Geometry: final body of the model. Coordinates: model frame, mm. A direction names the side the tool comes from. Give positions to 0.01 mm unless a question says otherwise; leave off trailing zeros. Loops run counter-clockwise (first coordinate to the right, second up) from the corner with the lowest first, then second, coordinate; pieces in that order, holes last.
1. Access query for faces 4 (the face through (53.24, -0.53, -11.99)), 5 (the face through (4.93, -18.17, 24.53)), 6 (the face through (135.357, 87.741, -3.252)), 7 (the face through (145.386, 68.872, -41.002)). Directions: +Z, -Z, +X, -X, +Y, -Y. A direction counts if a zero-diameter tool reaches every point of the face in a straight line with its end or side. Return the directions, or none.
2. Material intervals for line 1 along X through (y, z) = (108, 0); line 2 along Z through (x, y) = (70, 0); line 3 along Z through (x, y) = (210, 176), sorted ascending.
3. Section A-A, the plane y = 60. Output: boundary loops of the cut face in (x, z), then the cut area to 3 significant figures.
4. Draft query along Y for faces 1 (the face through (0, -8.3, 9.4)), 2 (the face through (238.394, 189.798, 141.033)), 3 (the face through (224.07, 177.95, 140.47)). Return one class per face: +Y half, -Y half, draft (parallel to the pull), parting line (faces both ways), or undercut.
5. First-contact query: P1, Ø19, axis at x = 150, z = 0, coming from the -Y side; P2, Ø3, axis at x = 153, z = -25.5, coming from the +Y side; P3, Ø14.5, axis at y = 0, z = 0, coming from the -X side. Flat tips, straight axial feed; report the tip coordinate or a pass-through.
from build123d import *

# Parameters (mm, degrees)
SWEEP_2_PROFILE_R    = 15
SWEEP_6_PROFILE_R    = 15
SKETCH_7_R           = 40
EXTRUDE_2_DEPTH      = 10
SKETCH_8_R           = 4.5
CUT_EXTRUDE_1_DEPTH  = 357.575052533
SWEEP_START          = 287.981272568
SWEEP_8_OUTLINE_R    = 45
SWEEP_8_DEPTH        = 12.094233032
SWEEP_START_2        = 300
SWEEP_8_2_OUTLINE_W  = 93
SWEEP_8_2_OUTLINE_H  = 93
SWEEP_8_2_DEPTH      = 1
EXTRUDE_3_REACH      = 435.125
EXTRUDE_3_END_RADIUS = 15
SKETCH_15_R          = 10
SWEEP_2_2_PROFILE_R  = 12
SWEEP_4_PROFILE_R    = 12
SKETCH_19_R          = 7
CUT_EXTRUDE_2_DEPTH  = 70
SWEEP_14_PROFILE_R   = 5.5
SWEEP_16_PROFILE_R   = 5.5
SWEEP_18_PROFILE_R   = 5.5
SWEEP_20_PROFILE_R   = 5.5


with BuildPart() as part:
    # Sweep 2: sweep along a path in 草图1
    with BuildLine(Plane.XY) as sweep_2_path:
        Line((0, 0), (105, 0))
        ThreePointArc((105, 0), (136.819805153, 13.180194847), (150, 45))
        Line((150, 45), (150, 77.56))
    # Sweep 2 profile (on start of the path) → Sweep 2 (sweep)
    with BuildSketch(Plane(origin=(0, 0, 0), x_dir=(0, 0, 1), z_dir=(1, 0, 0))):
        Circle(SWEEP_2_PROFILE_R)
    sweep(path=sweep_2_path.line)

    # 扫描6: sweep along a curve in space
    with BuildLine() as sweep_6_path:
        Line((150, 50, 0), (150, 120, 0))
        Line((150, 120, 0), (230, 200, 140))
    # 扫描6 profile (on start of the path) → 扫描6 (sweep)
    with BuildSketch(Plane(origin=(150, 50, 0), x_dir=(0, 0, 1), z_dir=(0, 1, 0))):
        Circle(SWEEP_6_PROFILE_R)
    sweep(path=sweep_6_path.line, transition=Transition.RIGHT)

    # 草图7 → 凸台-拉伸2 (add)
    with BuildSketch(Plane(origin=(0, 0, 0), x_dir=(0, 0, -1), z_dir=(1, 0, 0))):
        Circle(SKETCH_7_R)
    extrude(amount=EXTRUDE_2_DEPTH)

    # 草图8 → 切除-拉伸1 (cut, through all)
    with BuildSketch(Plane(origin=(0, 0, 0), x_dir=(0, 0, -1), z_dir=(1, 0, 0))):
        with Locations((-21.213203, 21.213203)):
            Circle(SKETCH_8_R)
        with Locations((21.213203, 21.213203)):
            Circle(SKETCH_8_R)
        with Locations((21.213203, -21.213203)):
            Circle(SKETCH_8_R)
        with Locations((-21.213203, -21.213203)):
            Circle(SKETCH_8_R)
    extrude(amount=CUT_EXTRUDE_1_DEPTH, mode=Mode.SUBTRACT)

    # 扫描8: read off the stored shape, not the designer's step
    # 扫描8 outline → 扫描8 (add)
    with BuildSketch(Plane(origin=(0, 0, 0), x_dir=(0.8956998912049878, -0.22074548276362646, -0.38599629108946926), z_dir=(0.4446590883984862, 0.4446590883984862, 0.7775323724509833)).offset(SWEEP_START)):
        with Locations((107.822397672, 104.113222554)):
            Circle(SWEEP_8_OUTLINE_R)
    extrude(amount=SWEEP_8_DEPTH)

    # Sweep 8 2 outline → Sweep 8 2 (cut)
    with BuildSketch(Plane(origin=(0, 0, 0), x_dir=(0.8958064164776169, -0.2205061948252594, -0.3858858409442036), z_dir=(0.4444444444444439, 0.4444444444444449, 0.7777777777777779)).offset(SWEEP_START_2)):
        with Locations((107.5, 104.5)):
            Rectangle(SWEEP_8_2_OUTLINE_W, SWEEP_8_2_OUTLINE_H)
    extrude(amount=SWEEP_8_2_DEPTH, mode=Mode.SUBTRACT)

    # 凸台-拉伸3: up to this cylinder (the profile starts outside it)
    extrude_3_end = Plane(origin=(150, 60, 0), z_dir=(0, 1, 0)) * Cylinder(EXTRUDE_3_END_RADIUS, 901.25, mode=Mode.PRIVATE)
    # 草图15 → 凸台-拉伸3 (add, up to the surface)
    with BuildSketch(Plane.XY.offset(-70), mode=Mode.PRIVATE) as extrude_3_sk1:
        with Locations(Location((150, 60, 0), (0, 0, 180))):
            Circle(SKETCH_15_R)
    extrude_3_tool1 = extrude(extrude_3_sk1.sketch, amount=EXTRUDE_3_REACH, mode=Mode.PRIVATE) - extrude_3_end
    add(extrude_3_tool1.solids().sort_by_distance((150, 60, -70))[0])

    # Sweep 2 2: sweep along a path in 草图16
    with BuildLine(Plane.XY) as sweep_2_2_path:
        Line((-10, 0), (105, 0))
        ThreePointArc((105, 0), (136.819805153, 13.180194847), (150, 45))
        Line((150, 45), (150, 77.56))
    # Sweep 2 2 profile (on start of the path) → Sweep 2 2 (sweep, cut)
    with BuildSketch(Plane(origin=(-10, 0, 0), x_dir=(0, 0, 1), z_dir=(1, 0, 0))):
        Circle(SWEEP_2_2_PROFILE_R)
    sweep(path=sweep_2_2_path.line, mode=Mode.SUBTRACT)

    # 切除-扫描4: sweep along a curve in space
    with BuildLine() as sweep_4_path:
        Line((150, 50, 0), (150, 120, 0))
        Line((150, 120, 0), (236.67, 206.67, 151.67))
    # 切除-扫描4 profile (on start of the path) → 切除-扫描4 (sweep, cut)
    with BuildSketch(Plane(origin=(150, 50, 0), x_dir=(0, 0, 1), z_dir=(0, 1, 0))):
        Circle(SWEEP_4_PROFILE_R)
    sweep(path=sweep_4_path.line, transition=Transition.RIGHT, mode=Mode.SUBTRACT)

    # 草图19 → 切除-拉伸2 (cut)
    with BuildSketch(Plane.XY.offset(-70)):
        with Locations(Location((150, 60, 0), (0, 0, 180))):
            Circle(SKETCH_19_R)
    extrude(amount=CUT_EXTRUDE_2_DEPTH, mode=Mode.SUBTRACT)

    # 切除-扫描14: sweep along a curve in space
    with BuildLine() as sweep_14_path:
        Line((262.842, 185.134, 149.017), (249.508, 171.8, 125.683))
    # 切除-扫描14 profile (on start of the path) → 切除-扫描14 (sweep, cut)
    with BuildSketch(Plane(origin=(262.842, 185.134, 149.017), x_dir=(-0.8682385624984269, 0, 0.4961469526165259), z_dir=(-0.4444502055235574, -0.4444502055235574, -0.7777711936168215))):
        Circle(SWEEP_14_PROFILE_R)
    sweep(path=sweep_14_path.line, mode=Mode.SUBTRACT)

    # 切除-扫描16: sweep along a curve in space
    with BuildLine() as sweep_16_path:
        Line((252.241, 228.2, 130.462), (238.907, 214.866, 107.128))
    # 切除-扫描16 profile (on start of the path) → 切除-扫描16 (sweep, cut)
    with BuildSketch(Plane(origin=(252.241, 228.2, 130.462), x_dir=(-0.868238562498427, 0, 0.4961469526165257), z_dir=(-0.4444502055235573, -0.4444502055235573, -0.7777711936168217))):
        Circle(SWEEP_16_PROFILE_R)
    sweep(path=sweep_16_path.line, mode=Mode.SUBTRACT)

    # 切除-扫描18: sweep along a curve in space
    with BuildLine() as sweep_18_path:
        Line((210.492, 228.2, 154.317), (197.158, 214.866, 130.983))
    # 切除-扫描18 profile (on start of the path) → 切除-扫描18 (sweep, cut)
    with BuildSketch(Plane(origin=(210.492, 228.2, 154.317), x_dir=(-0.8682385624984262, 0, 0.496146952616527), z_dir=(-0.44445020552355863, -0.44445020552355674, -0.7777711936168212))):
        Circle(SWEEP_18_PROFILE_R)
    sweep(path=sweep_18_path.line, mode=Mode.SUBTRACT)

    # 切除-扫描20: sweep along a curve in space
    with BuildLine() as sweep_20_path:
        Line((221.093, 185.134, 172.872), (207.759, 171.8, 149.538))
    # 切除-扫描20 profile (on start of the path) → 切除-扫描20 (sweep, cut)
    with BuildSketch(Plane(origin=(221.093, 185.134, 172.872), x_dir=(-0.8682385624984266, 0, 0.4961469526165266), z_dir=(-0.4444502055235583, -0.44445020552355635, -0.7777711936168216))):
        Circle(SWEEP_20_PROFILE_R)
    sweep(path=sweep_20_path.line, mode=Mode.SUBTRACT)


solid = part.part
Answers below:
1. face 4: -X
1. face 5: +X, -X
1. face 6: none
1. face 7: -Z
2. line 1: x = 135 to 138, 162 to 165
2. line 2: z = -15 to -12, 12 to 15
2. line 3: z = 78.06 to 82.94, 120.05 to 124.94, 163.64 to 165.14
3. outline: (140, -70) - (143, -70) - (143, -9.75) arc R12 cw (long way) to (157, -9.75) - (157, -70) - (160, -70) - (160, -11.18) arc R15 ccw (long way) to (140, -11.18) - close
3. area: 556 mm2
4. face 1: draft
4. face 2: +Y half
4. face 3: undercut
5. P1: stops at y = -3.37
5. P2: stops at y = 69.89
5. P3: stops at x = 127.78
